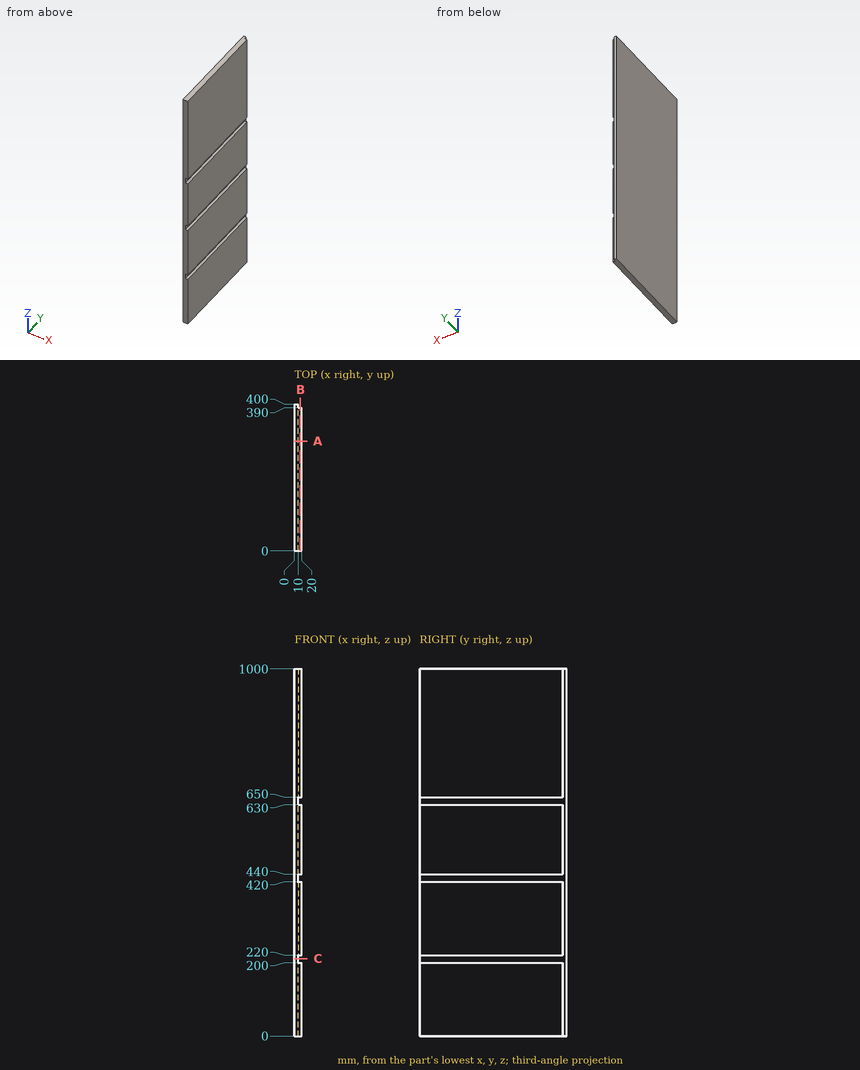
Answer from the drawing. Dimensions are ordinates in mm from the lowest x, y and z of the part. Coordinates: 2 decimals unless noted, no trailing zeros. Write each loop counter-clockwise with the first axis right and the second up, starting at its lowest first coordinate (ties: lowest second). Pieces come first, ordered by that corner, then holes. Notation, with made-up numbers: M 13,-29.75 L 42,-29.75 A6 ccw 42,-23.75 Z; hole C -32,51 d4. An arc over 180 degrees is marked long. Write item = value, one per line.
1. The part is cut by section C-C (z = 210.5). Determine the outline of the cut face in (x, y).
Solution:
outline = M 0,0 L 10,0 L 10,400 L 0,400 Z
2. The part is cut by section A-A (y = 299). Determine the outline of the cut face in (x, z), then the cut area to 3 significant figures.
Solution:
outline = M 0,0 L 20,0 L 20,200 L 10,200 L 10,220 L 20,220 L 20,420 L 10,420 L 10,440 L 20,440 L 20,630 L 10,630 L 10,650 L 20,650 L 20,1000 L 0,1000 Z
area = 19,400 mm2
3. A flat-ended cylindrical pin translates along its axis: pin 1 (5 mm diameter, centred on x = 13, z = 356.5, fed in from +Y). Find the tip coordinate at first contact, or state that the pin passes through.
Solution:
pin_1 = 390
4. The part is cut by section B-B (x = 16). Determine the outline of the cut face in (y, z).
Solution:
outline = M 0,0 L 390,0 L 390,200 L 0,200 Z; M 0,220 L 390,220 L 390,420 L 0,420 Z; M 0,440 L 390,440 L 390,630 L 0,630 Z; M 0,650 L 390,650 L 390,1000 L 0,1000 Z
5. Straight lines are drawn through the part: line 1 (Z direction, x = 16, y = 52); line 2 (Y direction, x = 17.75, z = 306.5). For each, find the intervals that lie inside material, in ascending order. Write a range as from..to.
Solution:
line_1 = 0..200, 220..420, 440..630, 650..1000
line_2 = 0..390
